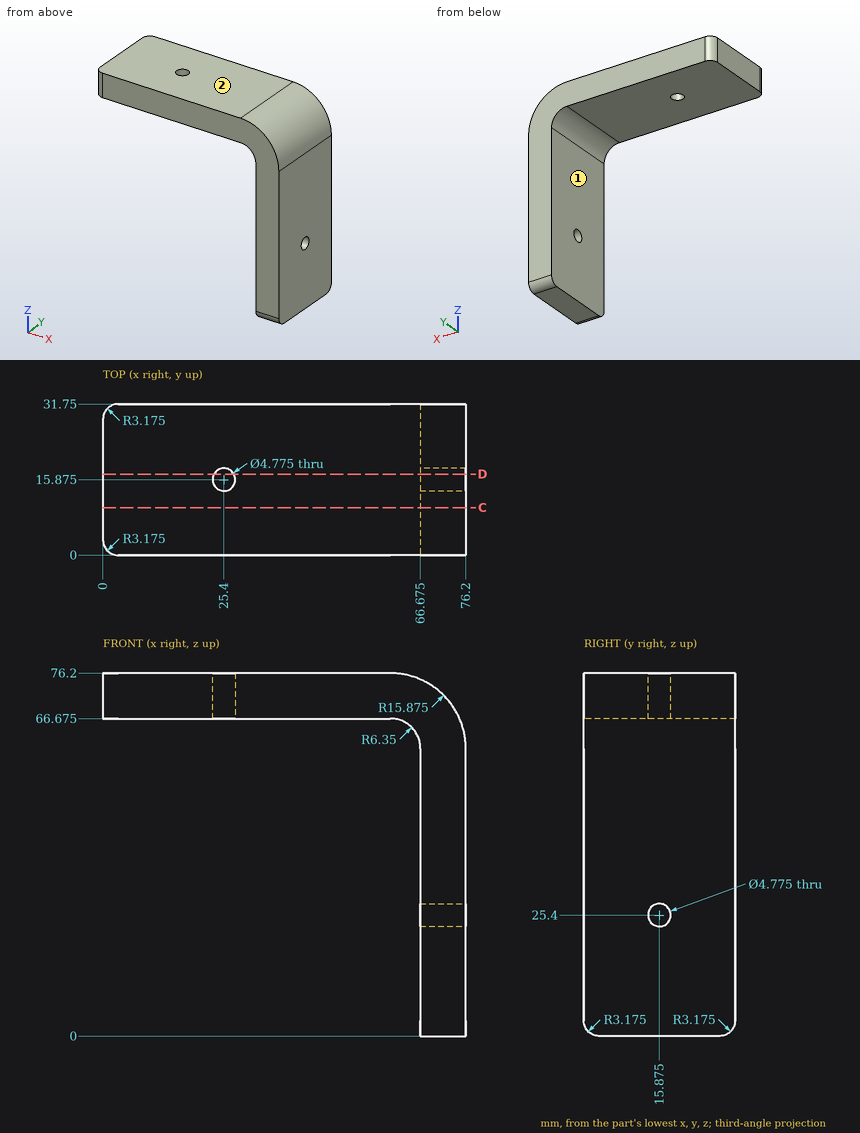
Answer from the drawing. Dimensions are ordinates in mm from the lowest x, y and z of the part. A direction names the side the tool comes from. Round coordinates to 2 decimals unless told otherwise and drop trailing zeros. Write each loop counter-clockwise with the first axis right and the second up, starting at its lowest first coordinate (ties: lowest second). Pieces come first, ordered by that corner, then holes. Notation, with made-up numbers: (21.5, 41) - (55.5, 41) arc R19 ccw to (55.5, 69) - close; hole circle Ø9 at (83, -1.5). An arc over 180 degrees is marked (long way). Use a Markdown table: item, result.
(1) Straight lines are drawn through the part: line 1 along Y through (x, z) = (25.4, 73); line 2 along X through (y, z) = (7, 3.5) (3 decimals). For each, find the intervals that lie inside material, in ascending order. Write a range as [from, to].
Reported:
| item | result |
|---|---|
| line 1 | [0, 13.49], [18.26, 31.75] |
| line 2 | [66.675, 76.2] |
(2) The part is cut by section D-D (y = 17). Write down the section's boundary in (x, z) (3 decimals).
Reported:
| item | result |
|---|---|
| outline | (0, 66.675) - (23.294, 66.675) - (23.294, 76.2) - (0, 76.2) - close; (27.506, 66.675) - (60.325, 66.675) arc R6.35 cw to (66.675, 60.325) - (66.675, 27.506) - (76.2, 27.506) - (76.2, 60.325) arc R15.875 ccw to (60.325, 76.2) - (27.506, 76.2) - close; (66.675, 0) - (76.2, 0) - (76.2, 23.294) - (66.675, 23.294) - close |
(3) Each of these flat-tipped pins is pushed along its axis until it touches: pin 1 Ø4 at (x, y) = (54, 25.5) entering from -Z (3 decimals); pin 2 Ø5 at (y, z) = (15.5, 51) entering from -X (3 decimals). Where does it stop, or does it pass through?
Reported:
| item | result |
|---|---|
| pin 1 | z = 66.675 |
| pin 2 | x = 66.675 |
(4) The part is cut by section C-C (y = 10). Write down the section's boundary in (x, z) (3 decimals).
Reported:
| item | result |
|---|---|
| outline | (0, 66.675) - (60.325, 66.675) arc R6.35 cw to (66.675, 60.325) - (66.675, 0) - (76.2, 0) - (76.2, 60.325) arc R15.875 ccw to (60.325, 76.2) - (0, 76.2) - close |
(5) Which of the six approach directions +Z, -Z, +X, -X, +Y, -Y give full straight-line access (tool end or side, diameter ignored) to the marked faces 1 and 2?
Reported:
| item | result |
|---|---|
| face 1 | -Z, -X, +Y, -Y |
| face 2 | +Z, +X, -X, +Y, -Y |
